```python
from build123d import *

# Parameters (mm, degrees)
SKETCH1_W           = 416.08
SKETCH1_H           = 101.6
BOSS_EXTRUDE2_DEPTH = 254
CUT_EXTRUDE1_DEPTH  = 101.6
CUT_EXTRUDE9_START  = 10.16
SKETCH6_W           = 187.48
SKETCH6_H           = 31.75
CUT_EXTRUDE9_DEPTH  = 244.84
SKETCH8_W           = 327.18
SKETCH8_H           = 12.7
CUT_EXTRUDE11_DEPTH = 228.6
CUT_EXTRUDE12_DEPTH = 417.08
CUT_EXTRUDE13_REACH = 65.5
SKETCH10_W          = 162.08
SKETCH10_H          = 13.204649201


with BuildPart() as part:
    # Sketch1 → Boss-Extrude2 (new body)
    with BuildSketch(Plane(origin=(0, 0, 0), x_dir=(1, 0, 0), z_dir=(0, 1, 0))):
        with Locations((208.04, 50.8)):
            Rectangle(SKETCH1_W, SKETCH1_H)
    extrude(amount=BOSS_EXTRUDE2_DEPTH)

    # Sketch2 → Cut-Extrude1 (cut)
    with BuildSketch(Plane.XY):
        Polygon((0, 101.6), (0, 254), (127, 254), align=None)
        Polygon((416.08, 254), (416.08, 101.6), (339.88, 254), align=None)
    extrude(amount=-CUT_EXTRUDE1_DEPTH, mode=Mode.SUBTRACT)

    # Sketch6 → Cut-Extrude9 (cut, through all)
    with BuildSketch(Plane(origin=(0, 0, 0), x_dir=(1, 0, 0), z_dir=(0, 1, 0)).offset(CUT_EXTRUDE9_START)):
        with Locations((233.44, 22.225)):
            Rectangle(SKETCH6_W, SKETCH6_H)
    extrude(amount=CUT_EXTRUDE9_DEPTH, mode=Mode.SUBTRACT)

    # Sketch8 → Cut-Extrude11 (cut)
    with BuildSketch(Plane(origin=(0, 254, 0), x_dir=(1, 0, 0), z_dir=(0, 1, 0))):
        with Locations((169.94, 50.8)):
            Rectangle(SKETCH8_W, SKETCH8_H)
        with Locations((169.94, 68.58)):
            Rectangle(SKETCH8_W, SKETCH8_H)
        with Locations((169.94, 86.36)):
            Rectangle(SKETCH8_W, SKETCH8_H)
    extrude(amount=-CUT_EXTRUDE11_DEPTH, mode=Mode.SUBTRACT)

    # Sketch9 → Cut-Extrude12 (cut, through all)
    with BuildSketch(Plane(origin=(416.08, 0, 0), x_dir=(0, 0, -1), z_dir=(1, 0, 0))):
        Polygon((0, 254), (0, 101.6), (38.1, 254), align=None)
    extrude(amount=-CUT_EXTRUDE12_DEPTH, mode=Mode.SUBTRACT)

    # Sketch10 → Cut-Extrude13 (cut, up to next)
    with BuildSketch(Plane.XY.offset(-38.1), mode=Mode.PRIVATE) as cut_extrude13_sk1:
        with Locations((233.44, 17.056383054)):
            Rectangle(SKETCH10_W, SKETCH10_H)
    cut_extrude13_tool1 = extrude(cut_extrude13_sk1.sketch, amount=-CUT_EXTRUDE13_REACH, mode=Mode.PRIVATE) & part.part
    add(cut_extrude13_tool1.solids().sort_by_distance((233.44, 17.056383, -38.1))[0], mode=Mode.SUBTRACT)


solid = part.part
```
Check sheet for the modelled part. Datum: model origin and axes. Units: mm. A direction names the side the tool comes from. Give positions to 0.01 mm unless a question says otherwise; leave off trailing zeros. Loops run counter-clockwise (first coordinate to the right, second up) from the corner with the lowest first, then second, coordinate; pieces in that order, holes last. Notation, with made-up numbers: M 32,-4 L 48,-4 A14 ccw 48,15 Z; hole C -5.75,35 d5. An arc over 180 degrees is marked long. Answer in a Markdown table with one row per item.
1) Cross-section at A-A (y = 30). Enter the section's corners in (x, z).
Solutions:
| item | result |
|---|---|
| outline | M 0,-101.6 L 416.08,-101.6 L 416.08,0 L 0,0 Z; hole M 6.35,-92.71 L 333.53,-92.71 L 333.53,-80.01 L 6.35,-80.01 Z; hole M 6.35,-74.93 L 333.53,-74.93 L 333.53,-62.23 L 6.35,-62.23 Z; hole M 6.35,-57.15 L 333.53,-57.15 L 333.53,-44.45 L 6.35,-44.45 Z; hole M 139.7,-38.1 L 327.18,-38.1 L 327.18,-6.35 L 139.7,-6.35 Z |
2) Cross-section at C-C (z = -87.5). Enter the section's corners in (x, y), plus the area to 3 significant figures.
Solutions:
| item | result |
|---|---|
| outline | M 0,0 L 416.08,0 L 416.08,101.6 L 339.88,254 L 333.53,254 L 333.53,25.4 L 6.35,25.4 L 6.35,109.22 L 0,101.6 Z; hole M 152.4,10.45 L 314.48,10.45 L 314.48,23.66 L 152.4,23.66 Z |
| area | 22,000 mm^2 |
3) Cross-section at D-D (x = 375.5). Enter the section's corners in (y, z).
Solutions:
| item | result |
|---|---|
| outline | M 0,-101.6 L 182.76,-101.6 L 182.76,-20.29 L 101.6,0 L 0,0 Z |
4) Tool access check on faces 4 (the face through (378.513, 176.733, -61.378)), 5 (the face through (232, 23.659, -69)), 6 (the face through (333.53, 141, -51)). Record the directions out of +Z, -Z, +X, -X, +Y, -Y that give a thin tool (end or side, any length) a straight path to the whole face; none if there is none.
Solutions:
| item | result |
|---|---|
| face 4 | +Z, -Z, +X, +Y |
| face 5 | -Z |
| face 6 | +Y |
5) Cross-section at B-B (x = 180). Enter the section's corners in (y, z), plus the area to 3 significant figures.
Solutions:
| item | result |
|---|---|
| outline | M 0,-101.6 L 10.45,-101.6 L 10.45,-38.1 L 10.16,-38.1 L 10.16,-6.35 L 127,-6.35 L 101.6,0 L 0,0 Z; M 23.66,-101.6 L 254,-101.6 L 254,-92.71 L 25.4,-92.71 L 25.4,-80.01 L 254,-80.01 L 254,-74.93 L 25.4,-74.93 L 25.4,-62.23 L 254,-62.23 L 254,-57.15 L 25.4,-57.15 L 25.4,-44.45 L 254,-44.45 L 254,-38.1 L 23.66,-38.1 Z |
| area | 7,630 mm^2 |
6) Depth check by flat-ended pin: pin 1 (16 mm diameter, centred on y = 167, z = -15, fed in from +X); pin 2 (2 mm diameter, centred on x = 146, z = -30.5, fed in from +Y); pin 3 (4 mm diameter, centred on y = 143, z = -51, fed in from -X). Enter the tip coordinate at first touch or a pass-through.
Solutions:
| item | result |
|---|---|
| pin 1 | stops at x = 387.38 |
| pin 2 | stops at y = 10.16 |
| pin 3 | stops at x = 333.53 |
7) Thickness scan on line 1 (Z direction, x = 203.5, y = 194); line 2 (X direction, y = 18, z = -83); line 3 (Y direction, x = 254.5, z = -95). Record the ranges inside material, lowest first.
Solutions:
| item | result |
|---|---|
| line 1 | z = -101.6 to -92.71, -80.01 to -74.93, -62.23 to -57.15, -44.45 to -38.1 |
| line 2 | x = 0 to 152.4, 314.48 to 416.08 |
| line 3 | y = 0 to 10.45, 23.66 to 254 |
8) Mould release check, pull along X, two halves, no side actions. Record for faces 1 (the face through (233, 254, -61)), 2 (the face through (0, 50, -50)), 3 (the face through (6.35, 68, -51)): released by +X, released by -X, zero draft, split by the parting line, or undercut.
Solutions:
| item | result |
|---|---|
| face 1 | zero draft |
| face 2 | released by -X |
| face 3 | undercut |
